Build history of the part. All positions in model axes, mm. Face numbers are marked on the shaded views. A direction names the side the tool comes from. Give positions to 0.01 mm unless a question says otherwise; leave off trailing zeros. Order: outer loops, then holes, each group sorted by start corner. A loop starts at its lowest first (then second) coordinate and runs counter-clockwise, first axis right, second up. Notation, with made-up numbers: M -6,-34 L 23,-34 A29 ccw 23,-8 Z; hole C -37.5,-34 d4. An arc over 180 degrees is marked long. One line per item, written item: value.
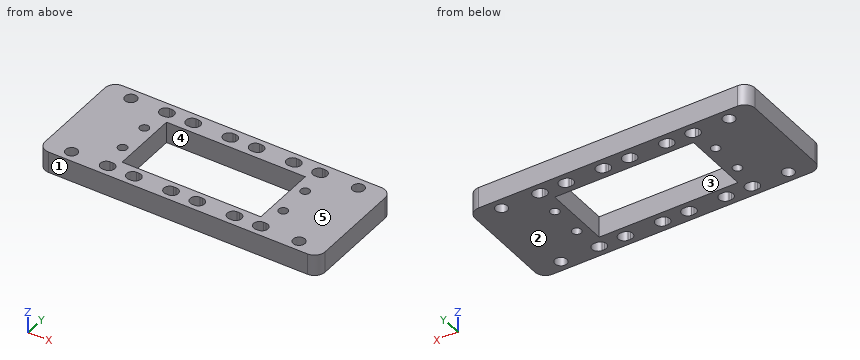
Autodesk Inventor part; units mm, degrees
ref_plane "YZ Plane" through (0, 0, 0) normal (1, 0, 0) x (0, 1, 0)
ref_plane "XZ Plane" through (0, 0, 0) normal (0, 1, 0) x (-1, 0, 0)
ref_plane "XY Plane" through (0, 0, 0) normal (0, 0, 1) x (1, 0, 0)
ref_plane "Work Plane1" through (0, 0, 0) normal (0, 0, 1) x (1, 0, 0)
sketch "Sketch2" plane through (0, 0, 0) normal (0, 0, 1) x (1, 0, 0)
  arc A0 (-24.5984, 11.6916) -> (-24.5984, 15.2476) centre (-24.5984, 13.4696) ccw
  line L0 (-24.5984, 15.2476) -> (-25.3604, 15.2476)
  line L1 (-25.3604, 11.6916) -> (-24.5984, 11.6916)
  arc A1 (-25.3604, 15.2476) -> (-25.3604, 11.6916) centre (-25.3604, 13.4696) ccw
  arc A2 (-25.3604, 15.2476) -> (-25.3604, 11.6916) centre (-25.3604, 13.4696) ccw
  arc A3 (-24.5984, 11.6916) -> (-24.5984, 15.2476) centre (-24.5984, 13.4696) ccw
  line L2 (-27.1384, 13.4696) -> (-22.8204, 13.4696) construction
  line L3 (-25.3604, 11.6916) -> (-24.5984, 11.6916)
  line L4 (-24.5984, 15.2476) -> (-25.3604, 15.2476)
  arc A4 (-25.3604, 15.2476) -> (-25.3604, 11.6916) centre (-25.3604, 13.4696) ccw
  arc A5 (-24.5984, 11.6916) -> (-24.5984, 15.2476) centre (-24.5984, 13.4696) ccw
  arc A6 (-33.2496, 15.2476) -> (-33.2496, 11.6916) centre (-33.2496, 13.4696) ccw
  arc A7 (-32.4876, 11.6916) -> (-32.4876, 15.2476) centre (-32.4876, 13.4696) ccw
  arc A8 (-43.6499, 11.6916) -> (-43.6499, 15.2476) centre (-43.6499, 13.4696) ccw
  arc A9 (-44.4119, 15.2476) -> (-44.4119, 11.6916) centre (-44.4119, 13.4696) ccw
  arc A10 (-51.5391, 11.6916) -> (-51.5391, 15.2476) centre (-51.5391, 13.4696) ccw
  arc A11 (-52.3011, 15.2476) -> (-52.3011, 11.6916) centre (-52.3011, 13.4696) ccw
  line L5 (-46.1899, 13.4696) -> (-41.8719, 13.4696) construction
  line L6 (-44.4119, 11.6916) -> (-43.6499, 11.6916)
  line L7 (-43.6499, 15.2476) -> (-44.4119, 15.2476)
  arc A12 (-44.4119, 15.2476) -> (-44.4119, 11.6916) centre (-44.4119, 13.4696) ccw
  arc A13 (-43.6499, 11.6916) -> (-43.6499, 15.2476) centre (-43.6499, 13.4696) ccw
  line L8 (-54.0791, 13.4696) -> (-49.7611, 13.4696) construction
  line L9 (-52.3011, 11.6916) -> (-51.5391, 11.6916)
  line L10 (-51.5391, 15.2476) -> (-52.3011, 15.2476)
  arc A14 (-52.3011, 15.2476) -> (-52.3011, 11.6916) centre (-52.3011, 13.4696) ccw
  arc A15 (-51.5391, 11.6916) -> (-51.5391, 15.2476) centre (-51.5391, 13.4696) ccw
  line L11 (-35.0276, 13.4696) -> (-30.7096, 13.4696) construction
  line L12 (-33.2496, 11.6916) -> (-32.4876, 11.6916)
  line L13 (-32.4876, 15.2476) -> (-33.2496, 15.2476)
  arc A16 (-33.2496, 15.2476) -> (-33.2496, 11.6916) centre (-33.2496, 13.4696) ccw
  arc A17 (-32.4876, 11.6916) -> (-32.4876, 15.2476) centre (-32.4876, 13.4696) ccw
  line L14 (-65.2414, 13.4696) -> (-60.9234, 13.4696) construction
  line L15 (-63.4634, 11.6916) -> (-62.7014, 11.6916)
  line L16 (-62.7014, 15.2476) -> (-63.4634, 15.2476)
  arc A18 (-63.4634, 15.2476) -> (-63.4634, 11.6916) centre (-63.4634, 13.4696) ccw
  arc A19 (-62.7014, 11.6916) -> (-62.7014, 15.2476) centre (-62.7014, 13.4696) ccw
  line L17 (-73.1307, 13.4696) -> (-68.8127, 13.4696) construction
  line L18 (-71.3527, 11.6916) -> (-70.5907, 11.6916)
  line L19 (-70.5907, 15.2476) -> (-71.3527, 15.2476)
  arc A20 (-71.3527, 15.2476) -> (-71.3527, 11.6916) centre (-71.3527, 13.4696) ccw
  arc A21 (-70.5907, 11.6916) -> (-70.5907, 15.2476) centre (-70.5907, 13.4696) ccw
  line L20 (-73.1307, -13.4696) -> (-68.8127, -13.4696) construction
  line L21 (-71.3527, -15.2476) -> (-70.5907, -15.2476)
  line L22 (-70.5907, -11.6916) -> (-71.3527, -11.6916)
  arc A22 (-71.3527, -11.6916) -> (-71.3527, -15.2476) centre (-71.3527, -13.4696) ccw
  arc A23 (-70.5907, -15.2476) -> (-70.5907, -11.6916) centre (-70.5907, -13.4696) ccw
  line L23 (-65.2414, -13.4696) -> (-60.9234, -13.4696) construction
  line L24 (-63.4634, -15.2476) -> (-62.7014, -15.2476)
  line L25 (-62.7014, -11.6916) -> (-63.4634, -11.6916)
  arc A24 (-63.4634, -11.6916) -> (-63.4634, -15.2476) centre (-63.4634, -13.4696) ccw
  arc A25 (-62.7014, -15.2476) -> (-62.7014, -11.6916) centre (-62.7014, -13.4696) ccw
  line L26 (-54.0791, -13.4696) -> (-49.7611, -13.4696) construction
  line L27 (-52.3011, -15.2476) -> (-51.5391, -15.2476)
  line L28 (-51.5391, -11.6916) -> (-52.3011, -11.6916)
  arc A26 (-52.3011, -11.6916) -> (-52.3011, -15.2476) centre (-52.3011, -13.4696) ccw
  arc A27 (-51.5391, -15.2476) -> (-51.5391, -11.6916) centre (-51.5391, -13.4696) ccw
  line L29 (-46.1899, -13.4696) -> (-41.8719, -13.4696) construction
  line L30 (-44.4119, -15.2476) -> (-43.6499, -15.2476)
  line L31 (-43.6499, -11.6916) -> (-44.4119, -11.6916)
  arc A28 (-44.4119, -11.6916) -> (-44.4119, -15.2476) centre (-44.4119, -13.4696) ccw
  arc A29 (-43.6499, -15.2476) -> (-43.6499, -11.6916) centre (-43.6499, -13.4696) ccw
  line L32 (-35.0276, -13.4696) -> (-30.7096, -13.4696) construction
  line L33 (-33.2496, -15.2476) -> (-32.4876, -15.2476)
  line L34 (-32.4876, -11.6916) -> (-33.2496, -11.6916)
  arc A30 (-33.2496, -11.6916) -> (-33.2496, -15.2476) centre (-33.2496, -13.4696) ccw
  arc A31 (-32.4876, -15.2476) -> (-32.4876, -11.6916) centre (-32.4876, -13.4696) ccw
  line L35 (-27.1384, -13.4696) -> (-22.8204, -13.4696) construction
  line L36 (-25.3604, -15.2476) -> (-24.5984, -15.2476)
  line L37 (-24.5984, -11.6916) -> (-25.3604, -11.6916)
  arc A32 (-25.3604, -11.6916) -> (-25.3604, -15.2476) centre (-25.3604, -13.4696) ccw
  arc A33 (-24.5984, -15.2476) -> (-24.5984, -11.6916) centre (-24.5984, -13.4696) ccw
  circle A34 centre (-72.1182, 4.953) radius 1.3525
  circle A35 centre (-72.1182, -4.953) radius 1.3525
  circle A36 centre (-23.8328, -4.953) radius 1.3525
  circle A37 centre (-23.8328, 4.953) radius 1.3525
  line L38 (-68.8127, 10.036) -> (-27.1475, 10.036)
  line L39 (-27.1475, 10.036) -> (-27.1475, -10.16)
  line L40 (-27.1475, -10.16) -> (-68.8127, -10.16)
  line L41 (-68.8127, -10.16) -> (-68.8127, 10.036)
  circle A38 centre (-81.7796, 13.4704) radius 1.778
  circle A39 centre (-81.7796, -13.4704) radius 1.778
  circle A40 centre (-81.7796, 13.4704) radius 1.778
  circle A41 centre (-81.7796, -13.4704) radius 1.778
  circle A42 centre (-13.4704, 13.4704) radius 1.778
  circle A43 centre (-13.4704, -13.4704) radius 1.778
  circle A44 centre (-13.4704, -13.4704) radius 1.778
  circle A45 centre (-13.4704, 13.4704) radius 1.778
  circle A46 centre (-89.6704, 13.4704) radius 1.778
  circle A47 centre (-89.6704, -13.4704) radius 1.778
  circle A48 centre (-5.5796, -13.4704) radius 1.778
  circle A49 centre (-5.5796, 13.4704) radius 1.778
  line L42 (-89.6704, 16.764) -> (-5.5796, 16.764)
  line L43 (-5.5796, 16.764) -> (-5.5796, -16.764)
  line L44 (-5.5796, -16.764) -> (-89.6704, -16.764)
  line L45 (-89.6704, -16.764) -> (-89.6704, 16.764)
  point P0 (0, 0)
  point P1 (-24.9794, 13.4696)
  point P2 (-44.0309, 13.4696)
  point P3 (-51.9201, 13.4696)
  point P4 (-32.8686, 13.4696)
  point P5 (-63.0824, 13.4696)
  point P6 (-70.9717, 13.4696)
  point P7 (-70.9717, -13.4696)
  point P8 (-63.0824, -13.4696)
  point P9 (-51.9201, -13.4696)
  point P10 (-44.0309, -13.4696)
  point P11 (-32.8686, -13.4696)
  point P12 (-24.9794, -13.4696)
extrude "Extrusion1" add sketch "Sketch2" along normal blind 6.35 contours A46 L45 | A46 L45 L42 L43 A49 A48 L44 A47 | A47 L45 | L43 A49 | L43 A48 picked at (-89.0777, 13.4704) picked at (-89.0777, -13.4704) picked at (-6.7028, 13.6737) picked at (-6.7028, -13.2671)
fillet "Fillet1" radius 3.175 4 edges at (-5.5796, 16.764, 3.175) (-89.6704, 16.764, 3.175) (-89.6704, -16.764, 3.175) (-5.5796, -16.764, 3.175)
properties part number "ExtendedServoMount"
1) Mould opens along Y. For the marked faces 1, 2 and 3 say: released by +Y, released by -Y, zero draft, split by the parting line, or undercut.
Check values:
face 1: released by -Y
face 2: zero draft
face 3: undercut
2) Saw through at D-D, the plane x = -81.5. Write the cut outline in (y, z).
Check values:
outline: M -16.76,0 L -15.23,0 L -15.23,6.35 L -16.76,6.35 Z; M -11.71,0 L 11.71,0 L 11.71,6.35 L -11.71,6.35 Z; M 15.23,0 L 16.76,0 L 16.76,6.35 L 15.23,6.35 Z
3) Saw through at C-C, the plane x = -64.5. Write the cut outline in (y, z).
Check values:
outline: M -16.76,0 L -14.91,0 L -14.91,6.35 L -16.76,6.35 Z; M -12.03,0 L -10.16,0 L -10.16,6.35 L -12.03,6.35 Z; M 10.04,0 L 12.03,0 L 12.03,6.35 L 10.04,6.35 Z; M 14.91,0 L 16.76,0 L 16.76,6.35 L 14.91,6.35 Z
4) Pin check, flat tip, straight feed: pin 1 (3 mm diameter, centred on x = -13.47, y = 13.47, fed in from +Z). Stop position of the tip, or through.
Check values:
pin 1: through
5) Drill centre lines: probe 1 along X at (y, z) = (-7, 1.75); probe 2 along Y at (x, z) = (-26, 2.5); probe 3 along X at (y, z) = (5.5, 3.5). Where is each one in solid material? Low to high. Write a range as from..to.
Check values:
probe 1: -89.67..-68.81, -27.15..-5.58
probe 2: -16.76..-15.13, -11.81..11.81, 15.13..16.76
probe 3: -89.67..-73.36, -70.88..-68.81, -27.15..-25.07, -22.6..-5.58
6) Saw through at A-A, the plane x = -49. Write the cut outline in (y, z).
Check values:
outline: M -16.76,0 L -10.16,0 L -10.16,6.35 L -16.76,6.35 Z; M 10.04,0 L 16.76,0 L 16.76,6.35 L 10.04,6.35 Z
7) Saw through at B-B, the plane y = -0.5. Write the cut outline in (x, z).
Check values:
outline: M -89.67,0 L -68.81,0 L -68.81,6.35 L -89.67,6.35 Z; M -27.15,0 L -5.58,0 L -5.58,6.35 L -27.15,6.35 Z
8) Tool access for the marked faces 4 and 5: list every direction of +Z, -Z, +X, -X, +Y, -Y with a clear straight run to the whole face (end or side of a thin tool).
Check values:
face 4: +Z, -Z
face 5: +Z, +X, -X, +Y, -Y
